Build history of the part. All positions in model axes, mm. A direction names the side the tool comes from. Give positions to 0.01 mm unless a question says otherwise; leave off trailing zeros. Order: outer loops, then holes, each group sorted by start corner. A loop starts at its lowest first (then second) coordinate and runs counter-clockwise, first axis right, second up. Notation, with made-up numbers: (-13, 47.25) - (13, 47.25) arc R28 cw to (13, 83.25) - close; hole circle Ø6 at (83, -40). An arc over 180 degrees is marked (long way). Use a Markdown table: item, result. Add a question column.
(1) Slice it at C-C (y = 0). Write the cut outline in (x, z), then the cut area to 3 significant figures.
(2) Slice it at D-D (z = 16.25). Write the cut outline in (x, y), then the cut area to 3 significant figures.
(3) Slice it at B-B (x = 7.25). Write the cut outline in (y, z), then the cut area to 3 significant figures.
(4) Mould opens along X. For faces 1 (the face through (3.754, -4.681, 20.814)), 2 (the face through (2.25, 1.99, 17.45)), 3 (the face through (-1.07, 0.82, 1.97)), 4 (the face through (0, 0, 4.836)) say: +X half, -X half, draft (parallel to the pull), parting line (faces both ways), or undercut.
(5) Flat gauge pins, fed straight in: pin 1 (2 mm diameter, centred on x = -0.5, y = -3, fed in from +Z); pin 2 (5 mm diameter, centred on y = 3.5, z = 1.5, fed in from +X); pin 3 (3 mm diameter, centred on x = 0, y = 0, fed in from -Z). Where does each tip first touch, or does it go through?
(6) Which spindle directions (+Z, -Z, +X, -X, +Y, -Y) get a long thin tool onto all of the face, cutting with end or side? Do faces 5 (the face through (-3.819, 4.628, -3.042)), 6 (the face through (-1.4, 0.7, 0)), 7 (the face through (-0.313, -1.313, 9.579)), 8 (the face through (-0.29, -1.32, 17.27)), 9 (the face through (-3.819, 4.628, 20.772)). Say none if no direction does.
(7) Wall check: line 1 (X direction, y = 0, z = 11); line 2 (Z direction, x = 3.25, y = -4.75); line 3 (Z direction, x = -5.75, y = 6). Give the ranges that are in metal, low to high.
(8) Slice it at A-A (z = 20.5). Write the cut outline in (x, y).
from build123d import *

# Parameters (mm, degrees)
SKETCH1_R           = 3
SKETCH1_R_2         = 1.35
BOSS_EXTRUDE1_DEPTH = 19.293356838
BOSS_EXTRUDE2_DEPTH = 6
CUT_EXTRUDE1_START  = -4
SKETCH3_R           = 1.35
CUT_EXTRUDE1_DEPTH  = 4
SKETCH4_R           = 1.35
CUT_EXTRUDE2_DEPTH  = 4


with BuildPart() as part:
    # Sketch1 → Boss-Extrude1 (new body)
    with BuildSketch(Plane.XY):
        Circle(SKETCH1_R)
        with Locations(Location((0, 0, 0), (0, 0, 39.125701285))):
            Circle(SKETCH1_R_2, mode=Mode.SUBTRACT)
    extrude(amount=BOSS_EXTRUDE1_DEPTH)

    # Sketch2 → Boss-Extrude2 (add)
    with BuildSketch(Plane(origin=(-2.327290276, -1.89307157, 0), x_dir=(0, 0, 1), z_dir=(-0.7757634254674072, -0.6310238566861593, 0))):
        Polygon((14.457294983, 3), (14.457294983, -3), (14.457294983, -9), (19.293356838, -9), (22.293356838, -9), (22.293356838, -6), (19.293356838, -6), (19.293356838, -3), (19.293356838, 3), (19.293356838, 6), (22.293356838, 6), (22.293356838, 9), (19.293356838, 9), (14.457294983, 9), align=None)
        Polygon((0, -9), (-3, -9), (-6, -9), (-6, -6), (-3, -6), (0, -6), (0, -3), (0, 3), (0, 6), (-3, 6), (-6, 6), (-6, 9), (-3, 9), (0, 9), (4.836061855, 9), (4.836061855, 3), (4.836061855, -3), (4.836061855, -9), align=None)
    extrude(amount=-BOSS_EXTRUDE2_DEPTH)

    # Sketch3 → Cut-Extrude1 (cut)
    with BuildSketch(Plane.XY.offset(19.293356838).offset(CUT_EXTRUDE1_START)):
        Circle(SKETCH3_R)
    extrude(amount=CUT_EXTRUDE1_DEPTH, mode=Mode.SUBTRACT)

    # Sketch4 → Cut-Extrude2 (cut)
    with BuildSketch(Plane(origin=(0, 0, 0), x_dir=(-1, 0, 0), z_dir=(0, 0, -1))):
        with Locations(Location((0, 0, 0), (0, 0, 180))):
            Circle(SKETCH4_R)
    extrude(amount=-CUT_EXTRUDE2_DEPTH, mode=Mode.SUBTRACT)


solid = part.part
Solution:
| question | item | result |
|---|---|---|
| 1 | outline | (-3.87, 0) - (-1.35, 0) - (-1.35, 4) - (1.35, 4) - (1.35, 0) - (3.87, 0) - (3.87, 4.84) - (3, 4.84) - (3, 14.46) - (3.87, 14.46) - (3.87, 19.29) - (1.35, 19.29) - (1.35, 15.29) - (-1.35, 15.29) - (-1.35, 19.29) - (-3.87, 19.29) - (-3.87, 14.46) - (-3, 14.46) - (-3, 4.84) - (-3.87, 4.84) - close; hole (-1.35, 4.84) - (1.35, 4.84) - (1.35, 14.46) - (-1.35, 14.46) - close |
| 1 | area | 85.0 mm2 |
| 2 | outline | (-8.01, 5.09) - (3.35, -8.87) - (8.01, -5.09) - (-3.35, 8.87) - close; hole circle Ø2.7 at (0, 0) |
| 2 | area | 102 mm2 |
| 3 | outline | (-5.7, -6) - (-4.16, -6) - (-4.16, 4.84) - (-5.7, 4.84) - close; (-5.7, 14.46) - (-4.16, 14.46) - (-4.16, 22.29) - (-5.7, 22.29) - close |
| 3 | area | 28.9 mm2 |
| 4 | face 1 | -X half |
| 4 | face 2 | +X half |
| 4 | face 3 | undercut |
| 4 | face 4 | undercut |
| 5 | pin 1 | z = 19.29 |
| 5 | pin 2 | x = 3.05 |
| 5 | pin 3 | z = 0 |
| 6 | face 5 | -Z, +X, -Y |
| 6 | face 6 | -Z |
| 6 | face 7 | none |
| 6 | face 8 | +Z |
| 6 | face 9 | +Z, +X, -Y |
| 7 | line 1 | -3 to -1.35, 1.35 to 3 |
| 7 | line 2 | 0 to 4.84, 14.46 to 19.29 |
| 7 | line 3 | -6 to 4.84, 14.46 to 22.29 |
| 8 | outline | (-8.01, 5.09) - (-6.11, 2.76) - (-1.46, 6.55) - (-3.35, 8.87) - close; (1.46, -6.55) - (3.35, -8.87) - (8.01, -5.09) - (6.11, -2.76) - close |
